The model under review builds one solid part; all positions refer to its coordinate system, in mm. A direction names the side the tool comes from. Coordinates: 2 decimals unless noted, no trailing zeros. Loops run counter-clockwise (first coordinate to the right, second up) from the corner with the lowest first, then second, coordinate; pieces in that order, holes last. Notation, with made-up numbers: (24, 57.25) - (48, 57.25) arc R24 ccw to (48, 91.25) - close; hole circle Ø8 at (86.25, -12). An arc over 180 degrees is marked (long way). One line per item, written item: value. Start each with the question number.
1. Mouldability with a two-part tool opening along Z and no side actions: class faces 4 (the face through (17.918, 51.495, 8.681)), 5 (the face through (56.825, 39.733, -0.791)), 6 (the face through (39.42, -0.25, 5.57)), 7 (the face through (39, 60.98, 0)) as +Z half, -Z half, draft (parallel to the pull), parting line (faces both ways), or undercut.
2. We need section B-B, the plane y = 46.5. Give the boundary of the cut face in (x, z), then the cut area to 3 significant figures.
3. We need section A-A, the plane y = 39. Give the boundary of the cut face in (x, z), then the cut area to 3 significant figures.
4. To check wall thickness, follow line 1 (X direction, y = 34, z = 0); line 2 (X direction, y = 44.5, z = 0); line 3 (Y direction, x = 35, z = 9.5). State the ranges of each line that lie inside material, in increasing order.
5. Insertion check: P1, Ø12, axis at x = 49, y = 9.5, coming from the +Z side; P2, Ø4, axis at x = 20, y = 28, coming from the -Z side; P3, Ø2, axis at y = 32.5, z = 30.5, coming from the -X side; P4, Ø13, axis at x = 38, z = -2, coming from the -Y side. Each pin has a flat end and moves straight along its axis. Give the tip position at first contact, or say it passes through.
6. For faces 1 (the face through (39, 18.888, -7)), 2 (the face through (48.11, 6.37, -3.84)), 3 (the face through (56, 42.272, 17)), list the 3-axis set-ups (+Z, -Z, +X, -X, +Y, -Y) from which the entire face can be reached by the end or side of a thin tool; tool diameter is ignored.
from build123d import *

# Parameters (mm, degrees)
F2_R     = 10.020621
F3_DEPTH = 25.4
F5_DEPTH = 12.7


with BuildPart() as f1:
    # F0 (on Top) → F1 (revolve)
    with BuildSketch(Plane.XY):
        Polygon((0, 42.272214), (0, 0), (20.86629, 28.241435), (20.86629, 50.906539), (32.378726, 50.906539), (32.378726, 18.887583), (38.854469, 18.887583), (38.854469, 60.979918), (16.189363, 60.979918), (16.189363, 42.272214), align=None)
    revolve(axis=Axis((38.854469, 39.93375, 0), (0, -1, 0)))

    # F2 (on face) → F3 (join)
    with BuildSketch(Plane.XZ.offset(-18.887583)):
        with Locations((38.854469, 0)):
            Circle(F2_R)
    extrude(amount=F3_DEPTH)

    # F4 (on face) → F5 (cut)
    with BuildSketch(Plane.XZ.offset(6.512417)):
        Polygon((32.418266, 0.59764), (35.118796, -5.275095), (41.554998, -5.872735), (45.290671, -0.59764), (42.590141, 5.275095), (36.153939, 5.872735), align=None)
    extrude(amount=-F5_DEPTH, mode=Mode.SUBTRACT)


solid = f1.part
Findings below:
1. face 4: parting line
1. face 5: undercut
1. face 6: undercut
1. face 7: draft
2. outline: circle Ø45.33 at (38.85, 0); circle Ø12.95 at (38.85, 0); hole circle Ø35.98 at (38.85, 0)
2. area: 729 mm2
3. outline: circle Ø77.71 at (38.85, 0); circle Ø12.95 at (38.85, 0); hole circle Ø35.98 at (38.85, 0)
3. area: 3,860 mm2
4. line 1: 0 to 20.87, 32.38 to 45.33, 56.84 to 77.71
4. line 2: 16.19 to 20.87, 32.38 to 45.33, 56.84 to 61.52
4. line 3: 50.91 to 60.98
5. P1: z = 38.63
5. P2: z = -35.01
5. P3: x = 13.57
5. P4: y = -6.51
6. face 1: none
6. face 2: -Y
6. face 3: +Y
